Design review of the part built by this model. Coordinates are the model's own, in mm. A direction names the side the tool comes from. Coordinates: 2 decimals unless noted, no trailing zeros. Write each loop counter-clockwise with the first axis right and the second up, starting at its lowest first coordinate (ties: lowest second). Pieces come first, ordered by that corner, then holes.
Q1. Mouldability with a two-part tool opening along X and no side actions: class faces 1 (the cylindrical face through (2.028, 6.536, 5.325)), 2 (the cylindrical face through (18.265, 1.268, 5.806)), 3 (the cylindrical face through (57.14, 2.03, 0.9)) as pulls with the +X half, pulls with the -X half, needs draft (parallel to the pull), parting line crosses it, or undercut.
Q2. Take a section at D-D (z = 1.25). Give the boundary of the cut face in (x, y), and give its area (3 significant figures).
Q3. Take a section at B-B (y = 12.25). Give the boundary of the cut face in (x, z), and give its area (3 significant figures).
Q4. For probe 1 along X at (y, z) = (9.25, 3.5); probe 2 along Y at (x, z) = (1.5, 5); probe 3 along X at (y, z) = (3.45, 5), list the stretches that pass through material, from the lowest coordinate up.
Q5. Take a section at C-C (z = 5). State how many separate pieces and enclosed holes the cut face has, and give its area (4 significant figures).
Q6. Take a section at A-A (x = 52). Give the boundary of the cut face in (y, z).
Q7. Insertion check: pin 1 (3 mm diameter, centred on x = 44, y = 4, fed in from +Z); pin 2 (3 mm diameter, centred on x = 27.5, z = 4.5, fed in from +Y); pin 3 (1.6 mm diameter, centred on x = 53.5, z = 5, fed in from +Y); pin 4 (5 mm diameter, centred on y = 9.5, z = 6.5, fed in from +X). Each pin has a flat end and moves straight along its axis. Give the tip position at first contact, or say it passes through.
Q8. Machinability: for faces 4 (the flat face through (55, 4, 5)), 5 (the flat face through (43, 3, 5)), 6 (the cylindrical face through (54.727, 3.26, 4.642)), 7 (the cylindrical face through (2.03, 12.1, 9.14)), 8 (the flat face through (0, 6, 5)), which of the approach directions +Z, -Z, +X, -X, +Y, -Y give a long, thin tool a straight path to every point of the face, cutting with its end or side? Answer none if there is none.
```python
from build123d import *

# Parameters (mm, degrees)
EXTRUDE_1_DEPTH     = 10
SKETCH_2_W          = 10
SKETCH_2_H          = 4
EXTRUDE_2_DEPTH     = 8
SKETCH_3_R          = 1.5
CUT_EXTRUDE_1_DEPTH = 5
SKETCH_4_R          = 2.75
CUT_EXTRUDE_2_DEPTH = 1.5
FILLET_1_R          = 3
SKETCH_5_R          = 1.5
CUT_EXTRUDE_3_DEPTH = 53.621288468
FILLET_2_R          = 3


with BuildPart() as part:
    # 草图1 → 凸台-拉伸1 (new body)
    with BuildSketch(Plane.XY):
        Polygon((0, 0), (0, 13), (4, 13), (4, 3), (10, 3), (10, 13), (14, 13), (14, 4), (36, 4), (36, 13), (40, 13), (40, 3), (46, 3), (46, 13), (50, 13), (50, 0), align=None)
    extrude(amount=EXTRUDE_1_DEPTH)

    # 草图2 → 凸台-拉伸2 (add)
    with BuildSketch(Plane(origin=(50, 0, 0), x_dir=(0, 0, -1), z_dir=(1, 0, 0))):
        with Locations((-5, 2)):
            Rectangle(SKETCH_2_W, SKETCH_2_H)
    extrude(amount=EXTRUDE_2_DEPTH)

    # 草图3 → 切除-拉伸1 (cut)
    with BuildSketch(Plane(origin=(0, 4, 0), x_dir=(1, 0, 0), z_dir=(0, 1, 0))):
        with Locations(Location((17, -5, 0), (0, 0, 270))):
            Circle(SKETCH_3_R)
        with Locations(Location((52, -5, 0), (0, 0, 270))):
            Circle(SKETCH_3_R)
    extrude(amount=-CUT_EXTRUDE_1_DEPTH, mode=Mode.SUBTRACT)

    # 草图4 → 切除-拉伸2 (cut)
    with BuildSketch(Plane(origin=(0, 4, 0), x_dir=(1, 0, 0), z_dir=(0, 1, 0))):
        with Locations(Location((17, -5, 0), (0, 0, 270))):
            Circle(SKETCH_4_R)
        with Locations(Location((52, -5, 0), (0, 0, 270))):
            Circle(SKETCH_4_R)
    extrude(amount=-CUT_EXTRUDE_2_DEPTH, mode=Mode.SUBTRACT)

    # 圆角1
    fillet_1_edges = [part.edges().sort_by_distance(p)[0] for p in [
        (48, 13, 10),
        (2, 13, 0),
        (12, 13, 0),
        (38, 13, 0),
        (48, 13, 0),
        (38, 13, 10),
        (12, 13, 10),
        (2, 13, 10),
    ]]
    fillet(fillet_1_edges, radius=FILLET_1_R)

    # 草图5 → 切除-拉伸3 (cut, through all)
    with BuildSketch(Plane(origin=(50, 0, 0), x_dir=(0, 0, -1), z_dir=(1, 0, 0))):
        with Locations((-5, 8)):
            Circle(SKETCH_5_R)
    extrude(amount=-CUT_EXTRUDE_3_DEPTH, mode=Mode.SUBTRACT)

    # 圆角2
    fillet_2_edges = [part.edges().sort_by_distance(p)[0] for p in [
        (58, 2, 10),
        (58, 2, 0),
    ]]
    fillet(fillet_2_edges, radius=FILLET_2_R)


solid = part.part
```
Response:
1. face 1: needs draft
1. face 2: undercut
1. face 3: pulls with the +X half
2. outline: (0, 0) - (57.44, 0) - (57.44, 4) - (50, 4) - (50, 12.44) - (46, 12.44) - (46, 3) - (40, 3) - (40, 12.44) - (36, 12.44) - (36, 4) - (14, 4) - (14, 12.44) - (10, 12.44) - (10, 3) - (4, 3) - (4, 12.44) - (0, 12.44) - close
2. area: 353 mm2
3. outline: (0, 1.02) - (4, 1.02) - (4, 8.98) - (0, 8.98) - close; (10, 1.02) - (14, 1.02) - (14, 8.98) - (10, 8.98) - close; (36, 1.02) - (40, 1.02) - (40, 8.98) - (36, 8.98) - close; (46, 1.02) - (50, 1.02) - (50, 8.98) - (46, 8.98) - close
3. area: 127 mm2
4. probe 1: x = 0 to 4, 10 to 14, 36 to 40, 46 to 50
4. probe 2: y = 0 to 6.5, 9.5 to 13
4. probe 3: x = 0 to 4, 10 to 14.25, 19.75 to 40, 46 to 49.25, 54.75 to 58
5. separate pieces: 7
5. enclosed holes: 0
5. area: 284.5 mm2
6. outline: (0, 0) - (4, 0) - (4, 2.25) - (2.5, 2.25) - (2.5, 3.5) - (0, 3.5) - close; (0, 6.5) - (2.5, 6.5) - (2.5, 7.75) - (4, 7.75) - (4, 10) - (0, 10) - close
7. pin 1: stops at z = 10
7. pin 2: stops at y = 4
7. pin 3: stops at y = 2.5
7. pin 4: stops at x = 50
8. face 4: +Z, -Z, +X, +Y
8. face 5: +Z, -Z, +Y
8. face 6: none
8. face 7: +Z, +X, -X, +Y
8. face 8: +Z, -Z, -X, +Y, -Y
